Here's the drawing with two shaded views (mm, measured from the low corner). I have some questions. Round coordinates to 2 decimals unless told otherwise and drop trailing zeros. Write each loop counter-clockwise with the first axis right and the second up, starting at its lowest first coordinate (ties: lowest second). Pieces come first, ordered by that corner, then holes. Notation, with made-up numbers: (34.5, -8) - (50.5, -8) arc R23 ccw to (50.5, 25) - close; hole circle Ø8 at (27.5, -8.75). An arc over 180 degrees is marked (long way). Return JSON: item names as keys, results as strings. Group by question number.
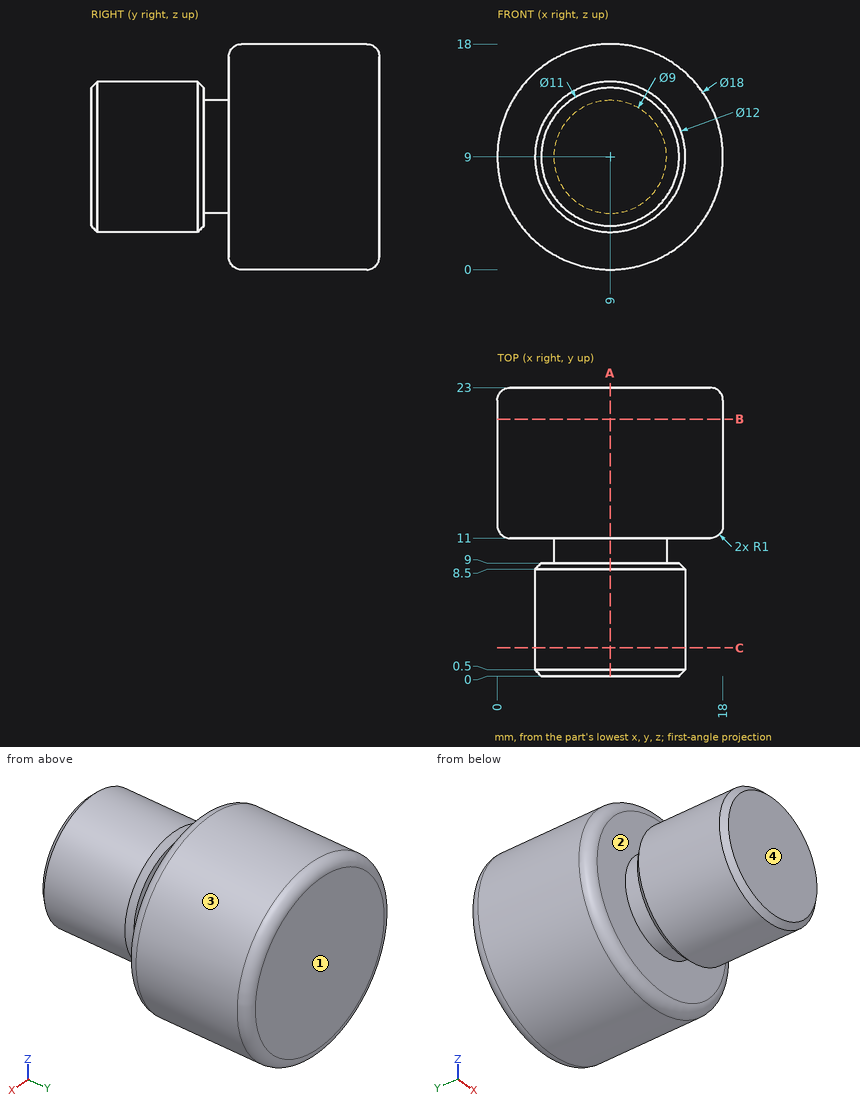
1) I need wall thicknesses on line 1 along Y through (x, z) = (4.5, 9.75); line 2 along Y through (x, z) = (10, 15); line 3 along Y through (x, z) = (13.5, 12.5). Which ranges of each line are inside material? Lowest first, please.
2) Imagine slicing it at A-A (x = 9). Please give me the cut outline in (y, z), plus the area to 3 significant figures.
3) If we mould it in two halves opening along Y, with no side actions, what happens to the marked faces 1, 2, 3 and 4? For each: released by +Y, released by -Y, zero draft, split by the parting line, or undercut.
4) Imagine slicing it at C-C (y = 2.25). Please give me the cut outline in (x, z), plus the area to 3 significant figures.
5) Will these pins go through, and if not, where does the flat tip stop? pin 1 Ø2 at (x, y) = (13.5, 6) entering from -Z; pin 2 Ø5 at (x, z) = (13, 15) entering from -Y; pin 3 Ø6 at (x, y) = (13, 14.5) entering from +Z; pin 4 Ø2 at (x, y) = (5, 17.5) entering from +Z.
6) Imagine slicing it at B-B (y = 20.5). Please give me the cut outline in (x, z), plus the area to 3 significant figures.
Results found:
{
 "1": {"line 1": "y = 0 to 9, 11 to 23", "line 2": "y = 11 to 23", "line 3": "y = 0.2 to 8.8, 11 to 23"},
 "2": {"outline": "(0, 3.5) - (0.5, 3) - (8.5, 3) - (9, 3.5) - (9, 4.5) - (11, 4.5) - (11, 1) arc R1 ccw to (12, 0) - (22, 0) arc R1 ccw to (23, 1) - (23, 17) arc R1 ccw to (22, 18) - (12, 18) arc R1 ccw to (11, 17) - (11, 13.5) - (9, 13.5) - (9, 14.5) - (8.5, 15) - (0.5, 15) - (0, 14.5) - close", "area": "341 mm²"},
 "3": {"face 1": "released by +Y", "face 2": "undercut", "face 3": "zero draft", "face 4": "released by -Y"},
 "4": {"outline": "circle Ø12 at (9, 9)", "area": "113 mm²"},
 "5": {"pin 1": "stops at z = 4.13", "pin 2": "stops at y = 0", "pin 3": "stops at z = 17.94", "pin 4": "stops at z = 17.49"},
 "6": {"outline": "circle Ø18 at (9, 9)", "area": "254 mm²"}
}
